from build123d import *

# Parameters (mm, degrees)
F0_W     = 520
F0_H     = 816
F1_DEPTH = 500
F2_W     = 360
F2_H     = 340
F3_DEPTH = 816.001
F4_W     = 656
F4_H     = 340
F5_DEPTH = 520.001


with BuildPart() as f1:
    # F0 (on Top) → F1 (new body)
    with BuildSketch(Plane.XY):
        Rectangle(F0_W, F0_H)
    extrude(amount=F1_DEPTH)

    # F2 (on face) → F3 (cut, through all)
    with BuildSketch(Plane(origin=(0, 408, 0), x_dir=(-1, 0, 0), z_dir=(0, 1, 0))):
        with Locations((0, 250)):
            Rectangle(F2_W, F2_H)
    extrude(amount=-F3_DEPTH, mode=Mode.SUBTRACT)

    # F4 (on face) → F5 (cut, through all)
    with BuildSketch(Plane(origin=(-260, 0, 0), x_dir=(0, -1, 0), z_dir=(-1, 0, 0))):
        with Locations((0, 250)):
            Rectangle(F4_W, F4_H)
    extrude(amount=-F5_DEPTH, mode=Mode.SUBTRACT)


solid = f1.part
Part model, mm, in its own coordinate system. A direction names the side the tool comes from. Coordinates: 2 decimals unless noted, no trailing zeros. Order: outer loops, then holes, each group sorted by start corner. A loop starts at its lowest first (then second) coordinate and runs counter-clockwise, first axis right, second up.
(1) Pull direction X, two halves, no side cores. Call faces 1 (the face through (-260, -5.7, 79.8)), 2 (the face through (-180, 369, 248)), 3 (the face through (219, 328, 248)): pulls with the +X half, pulls with the -X half, needs draft (parallel to the pull), parting line crosses it, or undercut.
Check sheet entries:
face 1: pulls with the -X half
face 2: undercut
face 3: needs draft
(2) Slice it at C-C, the plane y = -265. Write the cut outline in (x, z).
Check sheet entries:
outline: (-260, 0) - (260, 0) - (260, 80) - (-260, 80) - close; (-260, 420) - (260, 420) - (260, 500) - (-260, 500) - close
(3) Probe L1, parallel to Z at x = 77.5, y = -338.5; L2, parallel to Y at x = -230.5, z = 126; L3, parallel to X at y = -372.5, z = 253. List the from-to ranges inside material, lowest first.
Check sheet entries:
L1: z = 0 to 80, 420 to 500
L2: y = -408 to -328, 328 to 408
L3: x = -260 to -180, 180 to 260
(4) Slice it at B-B, the plane x = -106.5. Write the cut outline in (y, z).
Check sheet entries:
outline: (-408, 0) - (408, 0) - (408, 80) - (-408, 80) - close; (-408, 420) - (408, 420) - (408, 500) - (-408, 500) - close
(5) Tool access for faces 4 (the face through (-4, 6, 420)), 5 (the face through (180, 369, 248)), 6 (the face through (-3.6, 408, 79.8)), 7 (the face through (-221, -328, 248)): list every direction of +Z, -Z, +X, -X, +Y, -Y with a clear straight run to the whole face (end or side of a thin tool).
Check sheet entries:
face 4: none
face 5: +Y, -Y
face 6: +Z, -Z, +X, -X, +Y
face 7: +X, -X
(6) Slice it at A-A, the plane z = 179. Write the cut outline in (x, y), and give its area (3 significant figures).
Check sheet entries:
outline: (-260, -408) - (-180, -408) - (-180, -328) - (-260, -328) - close; (-260, 328) - (-180, 328) - (-180, 408) - (-260, 408) - close; (180, -408) - (260, -408) - (260, -328) - (180, -328) - close; (180, 328) - (260, 328) - (260, 408) - (180, 408) - close
area: 25,600 mm2
